Autodesk Inventor part; units mm, degrees
ref_plane "YZ Plane" through (0, 0, 0) normal (1, 0, 0) x (0, 1, 0)
ref_plane "XZ Plane" through (0, 0, 0) normal (0, 1, 0) x (-1, 0, 0)
ref_plane "XY Plane" through (0, 0, 0) normal (0, 0, 1) x (1, 0, 0)
sketch "Sketch1" plane through (0, 0, 0) normal (0, 1, 0) x (-1, 0, 0)
  line L0 (-20.3963, -7) -> (-20.3963, 13)
  line L1 (-20.3963, 15) -> (20.3963, 15)
  line L2 (20.3963, 13) -> (20.3963, -7)
  arc A0 (-20.3963, -7) -> (20.3963, -7) centre (0, -7) ccw
  line L3 (20.3963, 15) -> (30.3963, 15)
  line L4 (30.3963, 15) -> (30.3963, 13)
  line L5 (30.3963, 13) -> (20.3963, 13)
  line L6 (-20.3963, 15) -> (-30.3963, 15)
  line L7 (-30.3963, 15) -> (-30.3963, 13)
  line L8 (-30.3963, 13) -> (-20.3963, 13)
  point P0 (0, 0)
  point P1 (0, 15)
  point P2 (20.3963, 0)
  dimension "d1" = 2
  dimension "d2" = 2
  dimension "d3" = 10
  dimension "d4" = 10
  dimension "d5" = 20
  dimension "d6" = 20.3963
extrude "Extrusion1" add sketch "Sketch1" along normal mid plane 30
sketch "Sketch2" plane through (0, 15, 0) normal (0, 1, 0) x (1, 0, 0)
  line L0 (-15, 5.0963) -> (-10, 5.0963)
  line L1 (-10, 5.0963) -> (-10, 10.0963)
  line L2 (-10, 10.0963) -> (10, 10.0963)
  line L3 (10, 10.0963) -> (10, 5.0963)
  line L4 (10, 5.0963) -> (15, 5.0963)
  line L5 (15, 5.0963) -> (15, 7.3963)
  line L6 (15, 7.3963) -> (12.3, 7.3963)
  line L7 (12.3, 7.3963) -> (12.3, 12.3963)
  line L8 (12.3, 12.3963) -> (-12.3, 12.3963)
  line L9 (-12.3, 12.3963) -> (-12.3, 7.3963)
  line L10 (-12.3, 7.3963) -> (-15, 7.3963)
  line L11 (-15, 7.3963) -> (-15, 5.0963)
  arc A0 (20.3963, 7) -> (-20.3963, 7) centre (0, 7) ccw
  point P0 (0, 0)
  point P1 (0, 12.3963)
  point P2 (0, 10.0963)
  point P3 (0, 27.3963)
  point P4 (15, 6.2463)
  point P5 (-15, 6.2463)
  point P6 (10, 7.5963)
  point P7 (-10, 7.5963)
  point P8 (-12.5, 5.0963)
  point P9 (-13.65, 7.3963)
  dimension "d9" = 15
  dimension "d11" = 2.3
  dimension "d13" = 24.6
  dimension "d14" = 20
  dimension "d15" = 5
  dimension "d17" = 5
  dimension "d27" = 2.3
extrude "Extrusion2" cut sketch "Sketch2" against normal blind 25
sketch "Sketch3" plane through (30.3963, 15, 13) normal (0, 0, -1) x (-1, 0, 0)
  line L0 (0, -30) -> (0, 0)
  line L1 (0, 0) -> (10, 0)
  point P0 (30.3963, -15)
  point P1 (5, -15)
  point P2 (0, -15)
  point P3 (5, 0)
hole "Hole1" at (25.3963, 0, 13) direction (0, 0, 1) diameter 3 depth 2
mirror "Mirror1" about plane through (0, 0, 0) normal (1, 0, 0) of "Hole1"
properties part number "Part_B7"
Source: CAD feature listing. Evaluate the final solid. Frame: model axes, mm. A direction names the side the tool comes from. Round coordinates to 2 decimals unless told otherwise and drop trailing zeros. Loops run counter-clockwise (first coordinate to the right, second up) from the corner with the lowest first, then second, coordinate; pieces in that order, holes last. Notation, with made-up numbers: M -4.5,-7.75 L 24.5,-7.75 A13 cw 24.5,8.25 Z; hole C 13.25,34.5 d9. An arc over 180 degrees is marked long. Return JSON: item names as keys, results as strings. Group by question number.
1. Section query D-D on y = -12.25. Output: boundary loops of the cut face in (x, z), and give its area (3 significant figures).
2. Reachability of faces 1 (the face through (-28, 0, 13)), 2 (the face through (-12.3, 3, -10)), 3 (the face through (30.396, 0, 14)) from +Z, -Z, +X, -X, +Y, -Y: full face, straight path, thin tool, end or side. Return the list, or none.
3. Material intervals for line 1 along X through (y, z) = (-6, -7.5); line 2 along X through (y, z) = (0, 14); line 3 along Z through (x, y) = (-4.5, -0.25), sorted ascending. Write a range as from..to.
4. Section query B-B on y = 11.5. Output: boundary loops of the cut face in (x, z), and give its area (3 significant figures).
5. Pin query (flat end, axial travel): pin 1 (11 mm diameter, centred on x = 27, y = -6, fed in from -Z); pin 2 (3 mm diameter, centred on y = -5.5, z = -2, fed in from -X); pin 3 (6 mm diameter, centred on y = 1, z = -0.5, fed in from +X); pin 4 (2.5 mm diameter, centred on x = -25.4, y = 0, fed in from -Z). Return the tip coordinate at first contact, or that it passes through.
6. Mould query, pull axis X, two halves, no side actions, for faces 4 (the face through (20.396, 0, 3)), 5 (the face through (-23.932, -0.325, 14.014)), 6 (the face through (-30.396, 0, 14)). Classes: released by +X, released by -X, zero draft, split by the parting line, or undercut.
7. Section query C-C on z = -6. Output: boundary loops of the cut face in (x, y), and give its area (3 significant figures).
8. Section query A-A on y = 0. Output: boundary loops of the cut face in (x, z).
Checks:
{
 "1": {"outline": "M -30.4,13 L -20.4,13 L -20.4,-7 A20.4 ccw 20.4,-7 L 20.4,13 L 30.4,13 L 30.4,15 L -30.4,15 Z", "area": "1,590 mm²"},
 "2": {"face 1": "-Z, -X, +Y, -Y", "face 2": "+Y", "face 3": "+Z, -Z, +X, +Y, -Y"},
 "3": {"line 1": "x = -20.39..-12.3, -10..10, 12.3..20.39", "line 2": "x = -30.4..-26.9, -23.9..23.9, 26.9..30.4", "line 3": "z = -26.89..-12.4, -10.1..15"},
 "4": {"outline": "M -30.4,13 L -20.4,13 L -20.4,-7 A20.4 ccw 20.4,-7 L 20.4,13 L 30.4,13 L 30.4,15 L -30.4,15 Z; hole M -15,-7.4 L -12.3,-7.4 L -12.3,-12.4 L 12.3,-12.4 L 12.3,-7.4 L 15,-7.4 L 15,-5.1 L 10,-5.1 L 10,-10.1 L -10,-10.1 L -10,-5.1 L -15,-5.1 Z", "area": "1,500 mm²"},
 "5": {"pin 1": "stops at z = 13", "pin 2": "stops at x = -20.4", "pin 3": "stops at x = 20.4", "pin 4": "passes through"},
 "6": {"face 4": "released by +X", "face 5": "undercut", "face 6": "released by -X"},
 "7": {"outline": "M -20.4,-15 L 20.4,-15 L 20.4,15 L 15,15 L 15,-10 L 10,-10 L 10,15 L -10,15 L -10,-10 L -15,-10 L -15,15 L -20.4,15 Z", "area": "974 mm²"},
 "8": {"outline": "M -30.4,13 L -26.9,13 L -26.9,15 L -30.4,15 Z; M -23.9,13 L -20.4,13 L -20.4,-7 A20.4 ccw 20.4,-7 L 20.4,13 L 23.9,13 L 23.9,15 L -23.9,15 Z; M 26.9,13 L 30.4,13 L 30.4,15 L 26.9,15 Z; hole M -15,-7.4 L -12.3,-7.4 L -12.3,-12.4 L 12.3,-12.4 L 12.3,-7.4 L 15,-7.4 L 15,-5.1 L 10,-5.1 L 10,-10.1 L -10,-10.1 L -10,-5.1 L -15,-5.1 Z"}
}
